Print and shaded views of the part. All mm, measured from the part's lowest x, y and z. Coordinates: 2 decimals unless noted, no trailing zeros. Order: outer loops, then holes, each group sorted by start corner. A loop starts at its lowest first (then second) coordinate and runs counter-clockwise, first axis right, second up.
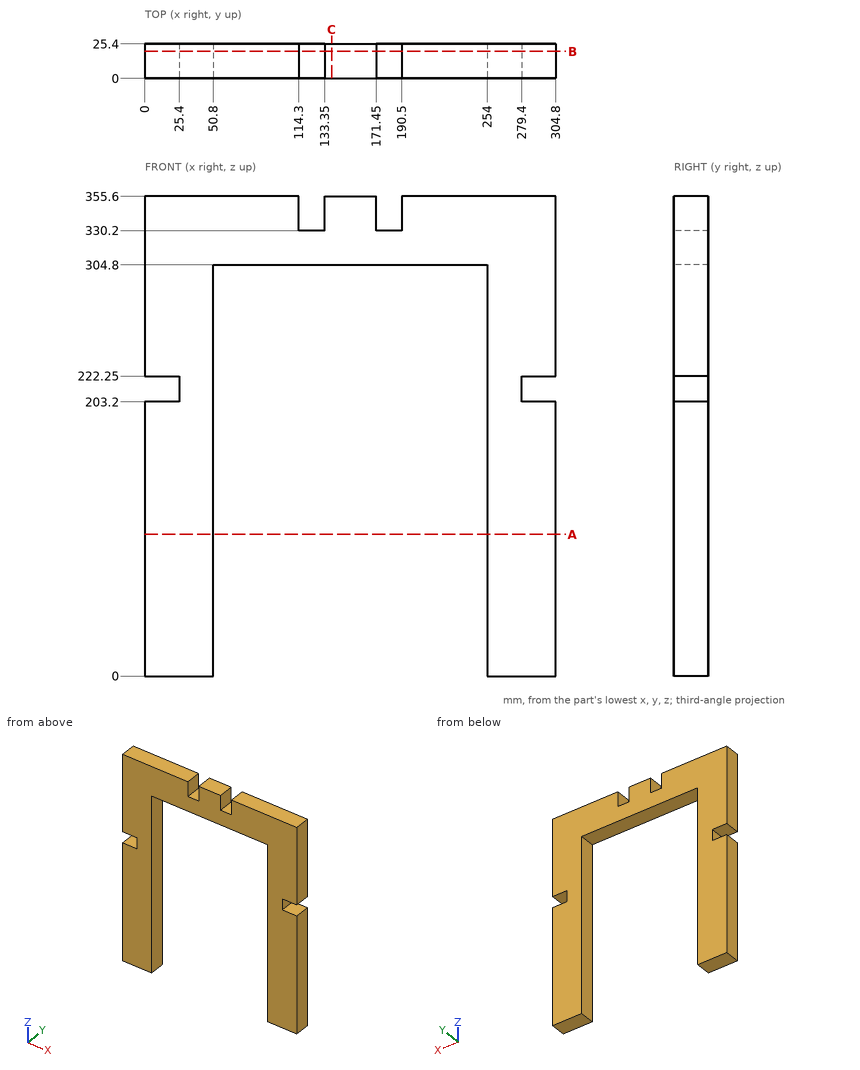
Q1. Cut at B-B, the plane y = 20. List the corners of the cut face in (x, z), plus the area to 3 significant figures.
Established:
outline: (0, 0) - (50.8, 0) - (50.8, 304.8) - (254, 304.8) - (254, 0) - (304.8, 0) - (304.8, 203.2) - (279.4, 203.2) - (279.4, 222.25) - (304.8, 222.25) - (304.8, 355.6) - (190.5, 355.6) - (190.5, 330.2) - (171.45, 330.2) - (171.45, 355.6) - (133.35, 355.6) - (133.35, 330.2) - (114.3, 330.2) - (114.3, 355.6) - (0, 355.6) - (0, 222.25) - (25.4, 222.25) - (25.4, 203.2) - (0, 203.2) - close
area: 44,500 mm2
Q2. Drop flat-ended pins along their axis: P1, Ø8, axis at x = 189, y = 20, coming from the -Z side; P2, Ø9.5, axis at y = 9.5, z = 212.5, coming from the -X side; P3, Ø15, axis at x = 125, y = 12, coming from the +Z side. Give the stop position or say it passes through.
Established:
P1: stops at z = 304.8
P2: stops at x = 25.4
P3: stops at z = 330.2
Q3. Cut at C-C, the plane x = 138.5. List the corners of the cut face in (y, z), plus the area to 3 significant figures.
Established:
outline: (0, 304.8) - (25.4, 304.8) - (25.4, 355.6) - (0, 355.6) - close
area: 1,290 mm2
Q4. Cut at A-A, the plane z = 105. List the corners of the cut face in (x, y), plus the area to 3 significant figures.
Established:
outline: (0, 0) - (50.8, 0) - (50.8, 25.4) - (0, 25.4) - close; (254, 0) - (304.8, 0) - (304.8, 25.4) - (254, 25.4) - close
area: 2,580 mm2
Q5. Probe line 1 (X direction, y = 13.5, z = 20); line 2 (X direction, y = 5.75, z = 206); line 3 (Z direction, x = 181, y = 21.75). List the from-to ranges inside material, lowest first.
Established:
line 1: x = 0 to 50.8, 254 to 304.8
line 2: x = 25.4 to 50.8, 254 to 279.4
line 3: z = 304.8 to 330.2
